The listing builds one solid part. Answer for the finished solid, in the listing's coordinates (mm). Give positions to 0.01 mm unless a question says otherwise; leave off trailing zeros. Order: outer loops, then holes, each group sorted by start corner. A loop starts at its lowest first (then second) coordinate and runs counter-clockwise, first axis right, second up.
```python
from build123d import *

# Parameters (mm, degrees)
SKETCH_1_W          = 150
SKETCH_1_H          = 230
EXTRUDE_1_DEPTH     = 3
CUT_EXTRUDE_1_REACH = 276.607
SKETCH_2_R          = 1.6
FILLET_1_R          = 4
CUT_EXTRUDE_2_REACH = 276.607
SKETCH_3_R          = 6
SKETCH_3_R_2        = 1.6
CUT_EXTRUDE_3_REACH = 276.607
SKETCH_4_R          = 1.6
SKETCH_4_R_2        = 3.25
SKETCH_4_W          = 7
SKETCH_4_H          = 14.5


with BuildPart() as part:
    # 草图1 → 凸台-拉伸1 (new body)
    with BuildSketch(Plane.XY):
        with Locations((75, 115)):
            Rectangle(SKETCH_1_W, SKETCH_1_H)
    extrude(amount=EXTRUDE_1_DEPTH)

    # 草图2 → 切除-拉伸1 (cut, up to next)
    with BuildSketch(Plane.XY.offset(3), mode=Mode.PRIVATE) as cut_extrude_1_sk1:
        with Locations((21.5, 8)):
            Circle(SKETCH_2_R)
    cut_extrude_1_tool1 = extrude(cut_extrude_1_sk1.sketch, amount=-CUT_EXTRUDE_1_REACH, mode=Mode.PRIVATE) & part.part
    # 草图2 → 切除-拉伸1 (cut, up to next)
    with BuildSketch(Plane.XY.offset(3), mode=Mode.PRIVATE) as cut_extrude_1_sk2:
        with Locations((47, 8)):
            Circle(SKETCH_2_R)
    cut_extrude_1_tool2 = extrude(cut_extrude_1_sk2.sketch, amount=-CUT_EXTRUDE_1_REACH, mode=Mode.PRIVATE) & part.part
    # 草图2 → 切除-拉伸1 (cut, up to next)
    with BuildSketch(Plane.XY.offset(3), mode=Mode.PRIVATE) as cut_extrude_1_sk3:
        with Locations((74.5, 10)):
            Circle(SKETCH_2_R)
    cut_extrude_1_tool3 = extrude(cut_extrude_1_sk3.sketch, amount=-CUT_EXTRUDE_1_REACH, mode=Mode.PRIVATE) & part.part
    # 草图2 → 切除-拉伸1 (cut, up to next)
    with BuildSketch(Plane.XY.offset(3), mode=Mode.PRIVATE) as cut_extrude_1_sk4:
        with Locations((145, 10)):
            Circle(SKETCH_2_R)
    cut_extrude_1_tool4 = extrude(cut_extrude_1_sk4.sketch, amount=-CUT_EXTRUDE_1_REACH, mode=Mode.PRIVATE) & part.part
    # 草图2 → 切除-拉伸1 (cut, up to next)
    with BuildSketch(Plane.XY.offset(3), mode=Mode.PRIVATE) as cut_extrude_1_sk5:
        with Locations((61.5, 180)):
            Circle(SKETCH_2_R)
    cut_extrude_1_tool5 = extrude(cut_extrude_1_sk5.sketch, amount=-CUT_EXTRUDE_1_REACH, mode=Mode.PRIVATE) & part.part
    # 草图2 → 切除-拉伸1 (cut, up to next)
    with BuildSketch(Plane.XY.offset(3), mode=Mode.PRIVATE) as cut_extrude_1_sk6:
        with Locations((145, 190)):
            Circle(SKETCH_2_R)
    cut_extrude_1_tool6 = extrude(cut_extrude_1_sk6.sketch, amount=-CUT_EXTRUDE_1_REACH, mode=Mode.PRIVATE) & part.part
    # 草图2 → 切除-拉伸1 (cut, up to next)
    with BuildSketch(Plane.XY.offset(3), mode=Mode.PRIVATE) as cut_extrude_1_sk7:
        with Locations((145, 170)):
            Circle(SKETCH_2_R)
    cut_extrude_1_tool7 = extrude(cut_extrude_1_sk7.sketch, amount=-CUT_EXTRUDE_1_REACH, mode=Mode.PRIVATE) & part.part
    # 草图2 → 切除-拉伸1 (cut, up to next)
    with BuildSketch(Plane.XY.offset(3), mode=Mode.PRIVATE) as cut_extrude_1_sk8:
        with Locations((7, 181)):
            Circle(SKETCH_2_R)
    cut_extrude_1_tool8 = extrude(cut_extrude_1_sk8.sketch, amount=-CUT_EXTRUDE_1_REACH, mode=Mode.PRIVATE) & part.part
    # 草图2 → 切除-拉伸1 (cut, up to next)
    with BuildSketch(Plane.XY.offset(3), mode=Mode.PRIVATE) as cut_extrude_1_sk9:
        with Locations((7, 175)):
            Circle(SKETCH_2_R)
    cut_extrude_1_tool9 = extrude(cut_extrude_1_sk9.sketch, amount=-CUT_EXTRUDE_1_REACH, mode=Mode.PRIVATE) & part.part
    add(cut_extrude_1_tool1.solids().sort_by_distance((21.5, 8, 3))[0], mode=Mode.SUBTRACT)
    add(cut_extrude_1_tool2.solids().sort_by_distance((47, 8, 3))[0], mode=Mode.SUBTRACT)
    add(cut_extrude_1_tool3.solids().sort_by_distance((74.5, 10, 3))[0], mode=Mode.SUBTRACT)
    add(cut_extrude_1_tool4.solids().sort_by_distance((145, 10, 3))[0], mode=Mode.SUBTRACT)
    add(cut_extrude_1_tool5.solids().sort_by_distance((61.5, 180, 3))[0], mode=Mode.SUBTRACT)
    add(cut_extrude_1_tool6.solids().sort_by_distance((145, 190, 3))[0], mode=Mode.SUBTRACT)
    add(cut_extrude_1_tool7.solids().sort_by_distance((145, 170, 3))[0], mode=Mode.SUBTRACT)
    add(cut_extrude_1_tool8.solids().sort_by_distance((7, 181, 3))[0], mode=Mode.SUBTRACT)
    add(cut_extrude_1_tool9.solids().sort_by_distance((7, 175, 3))[0], mode=Mode.SUBTRACT)

    # 圆角1
    fillet_1_edges = [part.edges().sort_by_distance(p)[0] for p in [
        (0, 230, 1.5),
        (150, 230, 1.5),
    ]]
    fillet(fillet_1_edges, radius=FILLET_1_R)

    # 草图3 → 切除-拉伸2 (cut, up to next)
    with BuildSketch(Plane.XY.offset(3), mode=Mode.PRIVATE) as cut_extrude_2_sk1:
        with Locations((8, 135)):
            Circle(SKETCH_3_R)
    cut_extrude_2_tool1 = extrude(cut_extrude_2_sk1.sketch, amount=-CUT_EXTRUDE_2_REACH, mode=Mode.PRIVATE) & part.part
    # 草图3 → 切除-拉伸2 (cut, up to next)
    with BuildSketch(Plane.XY.offset(3), mode=Mode.PRIVATE) as cut_extrude_2_sk2:
        with Locations((8, 119)):
            Circle(SKETCH_3_R)
    cut_extrude_2_tool2 = extrude(cut_extrude_2_sk2.sketch, amount=-CUT_EXTRUDE_2_REACH, mode=Mode.PRIVATE) & part.part
    # 草图3 → 切除-拉伸2 (cut, up to next)
    with BuildSketch(Plane.XY.offset(3), mode=Mode.PRIVATE) as cut_extrude_2_sk3:
        with Locations((8, 166.5)):
            Circle(SKETCH_3_R_2)
    cut_extrude_2_tool3 = extrude(cut_extrude_2_sk3.sketch, amount=-CUT_EXTRUDE_2_REACH, mode=Mode.PRIVATE) & part.part
    # 草图3 → 切除-拉伸2 (cut, up to next)
    with BuildSketch(Plane.XY.offset(3), mode=Mode.PRIVATE) as cut_extrude_2_sk4:
        with Locations((8, 147)):
            Circle(SKETCH_3_R_2)
    cut_extrude_2_tool4 = extrude(cut_extrude_2_sk4.sketch, amount=-CUT_EXTRUDE_2_REACH, mode=Mode.PRIVATE) & part.part
    # 草图3 → 切除-拉伸2 (cut, up to next)
    with BuildSketch(Plane.XY.offset(3), mode=Mode.PRIVATE) as cut_extrude_2_sk5:
        with BuildLine():
            Line((6.25, 153.8), (6.25, 159.7))
            ThreePointArc((6.25, 159.7), (8, 161.45), (9.75, 159.7))
            Line((9.75, 159.7), (9.75, 153.8))
            ThreePointArc((9.75, 153.8), (8, 152.05), (6.25, 153.8))
        make_face()
    cut_extrude_2_tool5 = extrude(cut_extrude_2_sk5.sketch, amount=-CUT_EXTRUDE_2_REACH, mode=Mode.PRIVATE) & part.part
    add(cut_extrude_2_tool1.solids().sort_by_distance((8, 135, 3))[0], mode=Mode.SUBTRACT)
    add(cut_extrude_2_tool2.solids().sort_by_distance((8, 119, 3))[0], mode=Mode.SUBTRACT)
    add(cut_extrude_2_tool3.solids().sort_by_distance((8, 166.5, 3))[0], mode=Mode.SUBTRACT)
    add(cut_extrude_2_tool4.solids().sort_by_distance((8, 147, 3))[0], mode=Mode.SUBTRACT)
    add(cut_extrude_2_tool5.solids().sort_by_distance((8, 156.75, 3))[0], mode=Mode.SUBTRACT)

    # 草图4 → 切除-拉伸3 (cut, up to next)
    with BuildSketch(Plane.XY.offset(3), mode=Mode.PRIVATE) as cut_extrude_3_sk1:
        with Locations((22, 120)):
            Circle(SKETCH_4_R)
    cut_extrude_3_tool1 = extrude(cut_extrude_3_sk1.sketch, amount=-CUT_EXTRUDE_3_REACH, mode=Mode.PRIVATE) & part.part
    # 草图4 → 切除-拉伸3 (cut, up to next)
    with BuildSketch(Plane.XY.offset(3), mode=Mode.PRIVATE) as cut_extrude_3_sk2:
        with Locations((22, 189.5)):
            Circle(SKETCH_4_R)
    cut_extrude_3_tool2 = extrude(cut_extrude_3_sk2.sketch, amount=-CUT_EXTRUDE_3_REACH, mode=Mode.PRIVATE) & part.part
    # 草图4 → 切除-拉伸3 (cut, up to next)
    with BuildSketch(Plane.XY.offset(3), mode=Mode.PRIVATE) as cut_extrude_3_sk3:
        with Locations((24.415, 173.5)):
            Circle(SKETCH_4_R_2)
    cut_extrude_3_tool3 = extrude(cut_extrude_3_sk3.sketch, amount=-CUT_EXTRUDE_3_REACH, mode=Mode.PRIVATE) & part.part
    # 草图4 → 切除-拉伸3 (cut, up to next)
    with BuildSketch(Plane.XY.offset(3), mode=Mode.PRIVATE) as cut_extrude_3_sk4:
        with Locations((24.415, 159.5)):
            Circle(SKETCH_4_R_2)
    cut_extrude_3_tool4 = extrude(cut_extrude_3_sk4.sketch, amount=-CUT_EXTRUDE_3_REACH, mode=Mode.PRIVATE) & part.part
    # 草图4 → 切除-拉伸3 (cut, up to next)
    with BuildSketch(Plane.XY.offset(3), mode=Mode.PRIVATE) as cut_extrude_3_sk5:
        with Locations((24.32, 135.55)):
            Rectangle(SKETCH_4_W, SKETCH_4_H)
    cut_extrude_3_tool5 = extrude(cut_extrude_3_sk5.sketch, amount=-CUT_EXTRUDE_3_REACH, mode=Mode.PRIVATE) & part.part
    # 草图4 → 切除-拉伸3 (cut, up to next)
    with BuildSketch(Plane.XY.offset(3), mode=Mode.PRIVATE) as cut_extrude_3_sk6:
        with Locations((32.62, 135.55)):
            Rectangle(SKETCH_4_W, SKETCH_4_H)
    cut_extrude_3_tool6 = extrude(cut_extrude_3_sk6.sketch, amount=-CUT_EXTRUDE_3_REACH, mode=Mode.PRIVATE) & part.part
    add(cut_extrude_3_tool1.solids().sort_by_distance((22, 120, 3))[0], mode=Mode.SUBTRACT)
    add(cut_extrude_3_tool2.solids().sort_by_distance((22, 189.5, 3))[0], mode=Mode.SUBTRACT)
    add(cut_extrude_3_tool3.solids().sort_by_distance((24.415, 173.5, 3))[0], mode=Mode.SUBTRACT)
    add(cut_extrude_3_tool4.solids().sort_by_distance((24.415, 159.5, 3))[0], mode=Mode.SUBTRACT)
    add(cut_extrude_3_tool5.solids().sort_by_distance((24.32, 135.55, 3))[0], mode=Mode.SUBTRACT)
    add(cut_extrude_3_tool6.solids().sort_by_distance((32.62, 135.55, 3))[0], mode=Mode.SUBTRACT)


solid = part.part
```
1) For a pull along X with two mould halves and no side action, classify faces 1 (the flat face through (74, 117, 0)), 2 (the cylindrical face through (22.02, 175.697, 1.521)) as +X half, -X half, draft (parallel to the pull), parting line (faces both ways), or undercut.
Geometry says:
face 1: draft
face 2: undercut
2) Straight lines are drawn through the part: probe 1 along Y at (x, z) = (145, 1.95); probe 2 along Y at (x, z) = (47, 1); probe 3 along X at (y, z) = (132.5, 2.85). For each, find the intervals that lie inside material, in ascending order.
Geometry says:
probe 1: y = 0 to 8.4, 11.6 to 168.4, 171.6 to 188.4, 191.6 to 230
probe 2: y = 0 to 6.4, 9.6 to 230
probe 3: x = 0 to 2.55, 13.45 to 20.82, 27.82 to 29.12, 36.12 to 150
3) Find section A-A (x = 32.5). Write down the section's boundary in (y, z), then the cut area to 4 significant figures.
Geometry says:
outline: (0, 0) - (128.3, 0) - (128.3, 3) - (0, 3) - close; (142.8, 0) - (230, 0) - (230, 3) - (142.8, 3) - close
area: 646.5 mm2
4) Find section B-B (z = 2.05). Count the separate pieces of the cut face and the enclosed holes in it, then the cut area to 3 significant figures.
Geometry says:
separate pieces: 1
enclosed holes: 20
area: 33,900 mm2
